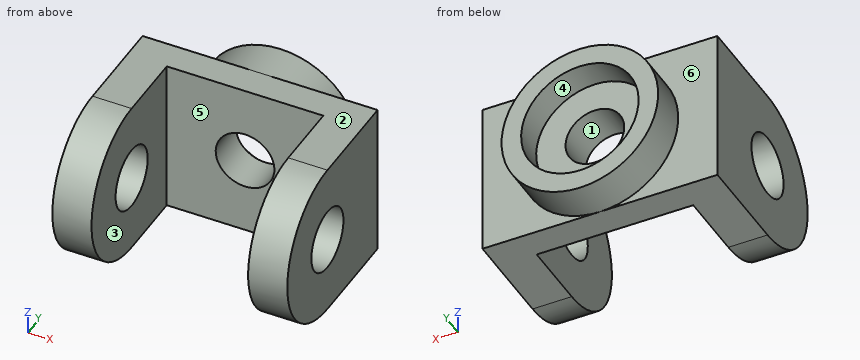
```python
from build123d import *

# Parameters (mm, degrees)
SKETCH1_W           = 120
SKETCH1_H           = 80
BOSS_EXTRUDE1_DEPTH = 15
SKETCH2_R           = 40
BOSS_EXTRUDE2_DEPTH = 20
SKETCH4_R           = 30
CUT_EXTRUDE1_DEPTH  = 15
SKETCH5_R           = 15
CUT_EXTRUDE2_DEPTH  = 42
SKETCH7_W           = 80
SKETCH7_H           = 35
BOSS_EXTRUDE3_DEPTH = 20
BOSS_EXTRUDE4_START = -20
SKETCH8_W           = 80
SKETCH8_H           = 35
BOSS_EXTRUDE4_DEPTH = 20
SKETCH9_R           = 16
CUT_EXTRUDE3_DEPTH  = 139


with BuildPart() as part:
    # Sketch1 → Boss-Extrude1 (new body)
    with BuildSketch(Plane(origin=(0, 0, 0), x_dir=(1, 0, 0), z_dir=(0, 1, 0))):
        Rectangle(SKETCH1_W, SKETCH1_H)
    extrude(amount=-BOSS_EXTRUDE1_DEPTH)

    # Sketch2 → Boss-Extrude2 (add)
    with BuildSketch(Plane(origin=(0, 0, 0), x_dir=(1, 0, 0), z_dir=(0, 1, 0))):
        with Locations(Location((0, 0, 0), (0, 0, 270))):
            Circle(SKETCH2_R)
    extrude(amount=BOSS_EXTRUDE2_DEPTH)

    # Sketch4 → Cut-Extrude1 (cut)
    with BuildSketch(Plane(origin=(0, 20, 0), x_dir=(1, 0, 0), z_dir=(0, 1, 0))):
        with Locations(Location((0, 0, 0), (0, 0, 270))):
            Circle(SKETCH4_R)
    extrude(amount=-CUT_EXTRUDE1_DEPTH, mode=Mode.SUBTRACT)

    # Sketch5 → Cut-Extrude2 (cut)
    with BuildSketch(Plane(origin=(0, 5, 0), x_dir=(1, 0, 0), z_dir=(0, 1, 0))):
        with Locations(Location((0, 0, 0), (0, 0, 270))):
            Circle(SKETCH5_R)
    extrude(amount=-CUT_EXTRUDE2_DEPTH, mode=Mode.SUBTRACT)

    # Sketch7 → Boss-Extrude3 (add)
    with BuildSketch(Plane(origin=(60, 0, 0), x_dir=(0, 0, -1), z_dir=(1, 0, 0))):
        with BuildLine():
            Line((-40, -50), (40, -50))
            ThreePointArc((40, -50), (0, -90), (-40, -50))
        make_face()
        with Locations((0, -32.5)):
            Rectangle(SKETCH7_W, SKETCH7_H)
    extrude(amount=-BOSS_EXTRUDE3_DEPTH)

    # Sketch8 → Boss-Extrude4 (add)
    with BuildSketch(Plane.ZY.offset(60).offset(BOSS_EXTRUDE4_START)):
        with BuildLine():
            Line((-40, -50), (40, -50))
            ThreePointArc((40, -50), (0, -90), (-40, -50))
        make_face()
        with Locations((0, -32.5)):
            Rectangle(SKETCH8_W, SKETCH8_H)
    extrude(amount=BOSS_EXTRUDE4_DEPTH)

    # Sketch9 → Cut-Extrude3 (cut)
    with BuildSketch(Plane.ZY.offset(60)):
        with Locations((0, -50)):
            Circle(SKETCH9_R)
    extrude(amount=-CUT_EXTRUDE3_DEPTH, mode=Mode.SUBTRACT)


solid = part.part
```
Source: CAD feature listing. Evaluate the final solid. Frame: model axes, mm. Face numbers are marked on the shaded views. A direction names the side the tool comes from. Round coordinates to 2 decimals unless told otherwise and drop trailing zeros. Write each loop counter-clockwise with the first axis right and the second up, starting at its lowest first coordinate (ties: lowest second). Pieces come first, ordered by that corner, then holes. Notation, with made-up numbers: M -2,50 L 15,50 A29 ccw 15,74 Z; hole C 81,67.25 d11. An arc over 180 degrees is marked long. Answer as a JSON object with one key per item and string values. Group by question number.
(1) Mould query, pull axis Z, two halves, no side actions, for the marked faces 1, 2 and 3. Classes: +Z half, -Z half, draft (parallel to the pull), parting line (faces both ways), or undercut.
(2) Section query A-A on y = -5.5. Output: boundary loops of the cut face in (x, z).
(3) Section query D-D on y = -76. Output: boundary loops of the cut face in (x, z), then the cut area to 3 significant figures.
(4) Reachability of the marked faces 4, 5 and 6 from +Z, -Z, +X, -X, +Y, -Y: full face, straight path, thin tool, end or side. Return the list, or none.
(5) First-contact query: pin 1 (3 mm diameter, centred on x = 34, y = 8.5, fed in from +Z); pin 2 (1.5 mm diameter, centred on x = -0.5, z = 29, fed in from +Y). Flat tips, straight axial feed; report the tip coordinate or a pass-through.
(6) Ray query, line 1 (X direction, y = -45.5, z = 28); line 2 (X direction, y = 12.5, z = 0); line 3 (Y direction, x = -15, z = 23). Return the intervals inside material, ascending. Write a range as [from, to].
(7) Section query C-C on x = 5. Output: boundary loops of the cut face in (y, z), then the cut area to 3 significant figures.
(8) Section query B-B on z = 0. Output: boundary loops of the cut face in (x, y), then the cut area to 3 significant figures.
Computed values:
{
 "1": {"face 1": "undercut", "face 2": "+Z half", "face 3": "draft"},
 "2": {"outline": "M -60,-40 L 60,-40 L 60,40 L -60,40 Z; hole C 0,0 d30"},
 "3": {"outline": "M -60,-30.4 L -40,-30.4 L -40,30.4 L -60,30.4 Z; M 40,-30.4 L 60,-30.4 L 60,30.4 L 40,30.4 Z", "area": "2,430 mm^2"},
 "4": {"face 4": "+Y", "face 5": "+Z, -Z, -Y", "face 6": "-X, +Y"},
 "5": {"pin 1": "z = 23.32", "pin 2": "y = 5"},
 "6": {"line 1": "[-60, -40], [40, 60]", "line 2": "[-40, -30], [30, 40]", "line 3": "[-15, 5]"},
 "7": {"outline": "M -15,-40 L 0,-40 L 0,-39.69 L 20,-39.69 L 20,-29.58 L 5,-29.58 L 5,-14.14 L -15,-14.14 Z; M -15,14.14 L 5,14.14 L 5,29.58 L 20,29.58 L 20,39.69 L 0,39.69 L 0,40 L -15,40 Z", "area": "1,330 mm^2"},
 "8": {"outline": "M -60,-90 L -40,-90 L -40,-66 L -60,-66 Z; M -60,-34 L -40,-34 L -40,-15 L -15,-15 L -15,5 L -30,5 L -30,20 L -40,20 L -40,0 L -60,0 Z; M 15,-15 L 40,-15 L 40,-34 L 60,-34 L 60,0 L 40,0 L 40,20 L 30,20 L 30,5 L 15,5 Z; M 40,-90 L 60,-90 L 60,-66 L 40,-66 Z", "area": "3,620 mm^2"}
}
